```python
from build123d import *

# Parameters (mm, degrees)
F2_DEPTH    = 3.556
F3_T1_DEPTH = 100.1960824302


# Not quite as in the source:
# - a fillet or chamfer that OpenCascade refuses, or shapes differently, is made with other operations: its cross-section is extruded or revolved along the edge and cut away or added


with BuildPart() as f2:
    # F1 (on offset) → F2 (new body)
    with BuildSketch(Plane.XZ.offset(-3.556)):
        with BuildLine():
            Line((-4.7608385794, 30.2790850401), (-4.7608385794, -3.7161211949))
            Line((-4.7608385794, -3.7161211949), (-2.9770701658, -5.2399407141))
            Line((-2.9770701658, -5.2399407141), (-2.9770701658, -17.5244603306))
            Line((-2.9770701658, -17.5244603306), (6.7130425275, -17.5824380662))
            Line((6.7130425275, -17.5824380662), (6.7868899709, -5.2399407141))
            Line((6.7868899709, -5.2399407141), (7.8166099265, -4.4050700963))
            Line((7.8166099265, -4.4050700963), (8.4343710914, -3.7950705737))
            Line((8.4343710914, -3.7950705737), (8.4343710914, 30.2790850401))
            add(Edge.make_bspline(
                [(-4.7608385794, 30.2790850401), (-4.5736827726, 31.9597863049), (-4.1702659217, 35.5825604162), (-1.8450394854, 41.296641728), (1.8526726795, 48.0701768841), (4.4004372394, 42.0002992607), (5.4469394771, 40.1971389087), (7.9610301665, 34.2093633894), (8.287935143, 31.4949825195), (8.4343710914, 30.2790850401)],
                knots=[0, 0, 0, 0, 0.1477315981, 0.3184374406, 0.4674111086, 0.6017993168, 0.7078404462, 0.869128143, 1, 1, 1, 1], degree=3))
        make_face()
    extrude(amount=F2_DEPTH)

    # F3: fillet of radius 26.3680405282 on 1 edges, made by hand

    # F3_s2 → F3_t1 (cut)
    with BuildSketch(Plane.XY.offset(-36.8560339819)):
        with BuildLine():
            ThreePointArc((8.4343710914, 3.556), (2.057056347, 0.904513961), (-4.7900142719, 0))
            Line((-4.7900142719, 0), (-4.7900142719, -0.5273608106))
            Line((-4.7900142719, -0.5273608106), (8.4343710914, -0.5273608106))
            Line((8.4343710914, -0.5273608106), (8.961731902, 0))
            ThreePointArc((8.961731902, 0), (8.961731902, 1.778), (8.6988587987, 3.0997591894))
            Line((8.6988587987, 3.0997591894), (8.4343710914, 3.556))
        make_face()
    extrude(amount=F3_T1_DEPTH, mode=Mode.SUBTRACT)


solid = f2.part
```
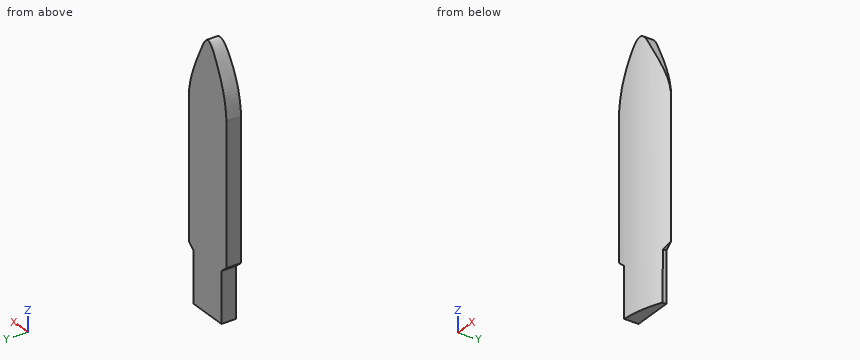
Design review of the part built by this model. Coordinates are the model's own, in mm. Give positions to 0.01 mm unless a question says otherwise; leave off trailing zeros. Loops run counter-clockwise (first coordinate to the right, second up) from the corner with the lowest first, then second, coordinate; pieces in that order, holes last. Notation, with made-up numbers: M 59,-12.5 L 65,-12.5 A29 ccw 65,19.5 Z; hole C 30,52 d2. An arc over 180 degrees is marked long. Return JSON: item names as keys, results as strings. Group by question number.
Item 1: We need section B-B (z = -10). Give the boundary of the cut face in (x, y).
Item 2: We need section A-A (z = 4). Give the boundary of the cut face in (x, y), and give its area (3 significant figures).
Item 3: For probe 1 along X at (y, z) = (3.35, -6.5); probe 2 along Z at (x, y) = (-0.5, 1); probe 3 along Y at (x, z) = (2.25, 34), list the stretches that pass through material, from the lowest coordinate up.
Item 4: Insertion check: pin 1 Ø1 at (y, z) = (2.5, -9.5) entering from -X; pin 2 Ø2 at (x, z) = (1, 30.5) entering from -Y; pin 3 Ø2 at (x, z) = (3, 25.5) entering from -Y. Each pin has a flat end and moves straight along its axis. Give the tip position at first contact, or say it passes through.
Output:
{
 "1": {"outline": "M -2.98,0.06 A26.37 ccw 6.76,2.66 L 6.76,3.56 L -2.98,3.56 Z"},
 "2": {"outline": "M -4.76,0 A26.37 ccw 8.43,3.56 L -4.76,3.56 Z", "area": "31.7 mm^2"},
 "3": {"probe 1": "x = -2.98 to 6.78", "probe 2": "z = -17.54 to 43.63", "probe 3": "y = 0.96 to 3.56"},
 "4": {"pin 1": "stops at x = -2.98", "pin 2": "stops at y = 0.44", "pin 3": "stops at y = 0.89"}
}
